Verification items for this drawing (mm, ordinates from the low corner). Coordinates: 2 decimals unless noted, no trailing zeros. Write each loop counter-clockwise with the first axis right and the second up, starting at its lowest first coordinate (ties: lowest second). Pieces come first, ordered by that corner, then holes. Notation, with made-up numbers: (49, 77.5) -> (97, 77.5) arc R18 ccw to (97, 105.5) -> close; hole circle Ø11 at (18, 65.25). An arc over 180 degrees is marked (long way). Put each result on its own line as item: value. Start each with the question number.
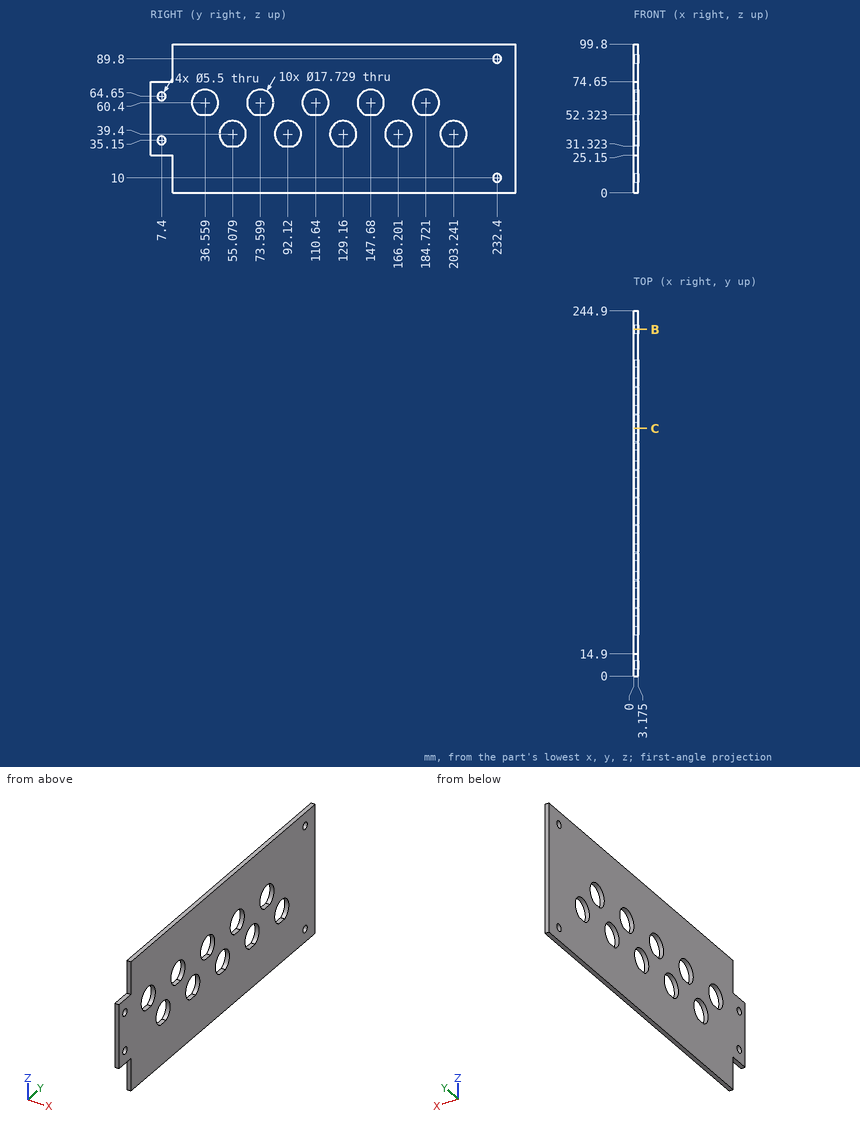
Item 1: Go/stop test with a flat-tipped pin: P1, Ø3.5, axis at y = 232.4, z = 10, coming from the -X side. Record where the tip stops, or that it passes through.
Item 2: Section check C-C, the plane y = 166. Enter the section's corners in (x, z) (1 decimal).
Item 3: Section check B-B, the plane y = 232.4. Give the number of separate pieces and of enclosed holes in the cut face, and give its area (3 significant figures).
Item 4: Scan lines: line 1 along Y through (x, z) = (1.55, 60.4) (1 decimal); line 2 along Z through (x, y) = (2.05, 232.4); line 3 along Y through (x, z) = (0.75, 39.4) (1 decimal). Record each from-to range of solid material in increasing order. Write a range as [from, to].
From the geometry:
1. P1: through
2. outline: (0, 0) -> (3.2, 0) -> (3.2, 31.3) -> (0, 31.3) -> close; (0, 48.3) -> (3.2, 48.3) -> (3.2, 99.8) -> (0, 99.8) -> close
3. separate pieces: 3
3. enclosed holes: 0
3. area: 282 mm²
4. line 1: [0, 27.7], [45.4, 64.7], [82.5, 101.8], [119.5, 138.8], [156.5, 175.9], [193.6, 244.9]
4. line 2: [0, 7.25], [12.75, 87.05], [92.55, 99.8]
4. line 3: [0, 46.2], [63.9, 83.3], [101, 120.3], [138, 157.3], [175.1, 194.4], [212.1, 244.9]
